from build123d import *

# Parameters (mm, degrees)
SKETCH1_R           = 125
SKETCH1_R_2         = 120
BOSS_EXTRUDE1_DEPTH = 10
SKETCH2_R           = 2.5
BOSS_EXTRUDE2_DEPTH = 100
SKETCH3_R           = 125
SKETCH3_R_2         = 120
BOSS_EXTRUDE3_DEPTH = 10
SKETCH4_R           = 2.5
BOSS_EXTRUDE4_DEPTH = 100
SKETCH5_R           = 125
SKETCH5_R_2         = 120
BOSS_EXTRUDE5_DEPTH = 10
SKETCH6_R           = 2.5
BOSS_EXTRUDE6_DEPTH = 100
SKETCH7_R           = 125
SKETCH7_R_2         = 120
BOSS_EXTRUDE7_DEPTH = 10
SKETCH8_R           = 2.5
BOSS_EXTRUDE8_DEPTH = 100
SKETCH9_R           = 125
SKETCH9_R_2         = 120
BOSS_EXTRUDE9_DEPTH = 10


with BuildPart() as part:
    # Sketch1 → Boss-Extrude1 (new body)
    with BuildSketch(Plane(origin=(0, 0, 0), x_dir=(1, 0, 0), z_dir=(0, 1, 0))):
        with Locations(Location((0, 0, 0), (0, 0, 270))):
            Circle(SKETCH1_R)
        with Locations(Location((0, 0, 0), (0, 0, 270))):
            Circle(SKETCH1_R_2, mode=Mode.SUBTRACT)
    extrude(amount=BOSS_EXTRUDE1_DEPTH)

    # Sketch2 → Boss-Extrude2 (add)
    with BuildSketch(Plane(origin=(0, 10, 0), x_dir=(1, 0, 0), z_dir=(0, 1, 0))):
        with Locations(Location((0, 122.5, 0), (0, 0, 270))):
            Circle(SKETCH2_R)
        with Locations(Location((106.088111964, 61.25, 0), (0, 0, 30))):
            Circle(SKETCH2_R)
        with Locations(Location((106.088111964, -61.25, 0), (0, 0, 150))):
            Circle(SKETCH2_R)
        with Locations(Location((0, -122.5, 0), (0, 0, 270))):
            Circle(SKETCH2_R)
        with Locations(Location((-106.088111964, -61.25, 0), (0, 0, 30))):
            Circle(SKETCH2_R)
        with Locations(Location((-106.088111964, 61.25, 0), (0, 0, 150))):
            Circle(SKETCH2_R)
    extrude(amount=BOSS_EXTRUDE2_DEPTH)

    # Sketch3 → Boss-Extrude3 (add)
    with BuildSketch(Plane(origin=(0, 110, 0), x_dir=(1, 0, 0), z_dir=(0, 1, 0))):
        with Locations(Location((0, 0, 0), (0, 0, 270))):
            Circle(SKETCH3_R)
        with Locations(Location((0, 0, 0), (0, 0, 270))):
            Circle(SKETCH3_R_2, mode=Mode.SUBTRACT)
    extrude(amount=BOSS_EXTRUDE3_DEPTH)

    # Sketch4 → Boss-Extrude4 (add)
    with BuildSketch(Plane(origin=(0, 120, 0), x_dir=(1, 0, 0), z_dir=(0, 1, 0))):
        with Locations(Location((0, 122.5, 0), (0, 0, 90))):
            Circle(SKETCH4_R)
        with Locations(Location((106.088111964, 61.25, 0), (0, 0, 30))):
            Circle(SKETCH4_R)
        with Locations(Location((106.088111964, -61.25, 0), (0, 0, 150))):
            Circle(SKETCH4_R)
        with Locations(Location((0, -122.5, 0), (0, 0, 90))):
            Circle(SKETCH4_R)
        with Locations(Location((-106.088111964, -61.25, 0), (0, 0, 30))):
            Circle(SKETCH4_R)
        with Locations(Location((-106.088111964, 61.25, 0), (0, 0, 150))):
            Circle(SKETCH4_R)
    extrude(amount=BOSS_EXTRUDE4_DEPTH)

    # Sketch5 → Boss-Extrude5 (add)
    with BuildSketch(Plane(origin=(0, 220, 0), x_dir=(1, 0, 0), z_dir=(0, 1, 0))):
        with Locations(Location((0, 0, 0), (0, 0, 270))):
            Circle(SKETCH5_R)
        with Locations(Location((0, 0, 0), (0, 0, 270))):
            Circle(SKETCH5_R_2, mode=Mode.SUBTRACT)
    extrude(amount=BOSS_EXTRUDE5_DEPTH)

    # Sketch6 → Boss-Extrude6 (add)
    with BuildSketch(Plane(origin=(0, 230, 0), x_dir=(1, 0, 0), z_dir=(0, 1, 0))):
        with Locations(Location((0, 122.5, 0), (0, 0, 90))):
            Circle(SKETCH6_R)
        with Locations(Location((106.088111964, 61.25, 0), (0, 0, 30))):
            Circle(SKETCH6_R)
        with Locations(Location((106.088111964, -61.25, 0), (0, 0, 150))):
            Circle(SKETCH6_R)
        with Locations(Location((0, -122.5, 0), (0, 0, 90))):
            Circle(SKETCH6_R)
        with Locations(Location((-106.088111964, -61.25, 0), (0, 0, 30))):
            Circle(SKETCH6_R)
        with Locations(Location((-106.088111964, 61.25, 0), (0, 0, 150))):
            Circle(SKETCH6_R)
    extrude(amount=BOSS_EXTRUDE6_DEPTH)

    # Sketch7 → Boss-Extrude7 (add)
    with BuildSketch(Plane(origin=(0, 330, 0), x_dir=(1, 0, 0), z_dir=(0, 1, 0))):
        with Locations(Location((0, 0, 0), (0, 0, 270))):
            Circle(SKETCH7_R)
        with Locations(Location((0, 0, 0), (0, 0, 270))):
            Circle(SKETCH7_R_2, mode=Mode.SUBTRACT)
    extrude(amount=BOSS_EXTRUDE7_DEPTH)

    # Sketch8 → Boss-Extrude8 (add)
    with BuildSketch(Plane(origin=(0, 340, 0), x_dir=(1, 0, 0), z_dir=(0, 1, 0))):
        with Locations(Location((0, 122.5, 0), (0, 0, 90))):
            Circle(SKETCH8_R)
        with Locations(Location((106.088111964, 61.25, 0), (0, 0, 30))):
            Circle(SKETCH8_R)
        with Locations(Location((106.088111964, -61.25, 0), (0, 0, 150))):
            Circle(SKETCH8_R)
        with Locations(Location((0, -122.5, 0), (0, 0, 90))):
            Circle(SKETCH8_R)
        with Locations(Location((-106.088111964, -61.25, 0), (0, 0, 30))):
            Circle(SKETCH8_R)
        with Locations(Location((-106.088111964, 61.25, 0), (0, 0, 150))):
            Circle(SKETCH8_R)
    extrude(amount=BOSS_EXTRUDE8_DEPTH)

    # Sketch9 → Boss-Extrude9 (add)
    with BuildSketch(Plane(origin=(0, 440, 0), x_dir=(1, 0, 0), z_dir=(0, 1, 0))):
        with Locations(Location((0, 0, 0), (0, 0, 270))):
            Circle(SKETCH9_R)
        with Locations(Location((0, 0, 0), (0, 0, 270))):
            Circle(SKETCH9_R_2, mode=Mode.SUBTRACT)
    extrude(amount=BOSS_EXTRUDE9_DEPTH)


solid = part.part
The listing builds one solid part. Answer for the finished solid, in the listing's coordinates (mm). Give positions to 0.01 mm unless a question says otherwise; leave off trailing zeros. Loops run counter-clockwise (first coordinate to the right, second up) from the corner with the lowest first, then second, coordinate; pieces in that order, holes last. Notation, with made-up numbers: (75.25, 84) - (103.25, 84) arc R20 ccw to (103.25, 101) - close; hole circle Ø4 at (-21, 18). An arc over 180 degrees is marked (long way). Write each question's results on one line, items separated by ' | '.
1. Find section B-B, the plane z = 0. Count the separate pieces of the cut face and the enclosed holes in it, then the cut area to 3 significant figures.
Resolved:
separate pieces: 10 | enclosed holes: 0 | area: 500 mm^2
2. Find section A-A, the plane y = 395. Write down the section's boundary in (x, z).
Resolved:
outline: circle Ø5 at (-106.09, -61.25); circle Ø5 at (-106.09, 61.25); circle Ø5 at (0, -122.5); circle Ø5 at (0, 122.5); circle Ø5 at (106.09, -61.25); circle Ø5 at (106.09, 61.25)
3. Consider probe 1 along X at (y, z) = (225, 0); probe 2 along X at (y, z) = (355.5, 60.5); probe 3 along Z at (x, y) = (1, 70.5). Determine where each line is inside the solid, lowest interval first. Write a range as from..to.
Resolved:
probe 1: x = -125..-120, 120..125 | probe 2: x = -108.47..-103.7, 103.7..108.47 | probe 3: z = -124.79..-120.21, 120.21..124.79
4. For a pull along Z with two mould halves and no side action, classify faces 1 (the face through (5.276, 334.93, -119.884)), 2 (the face through (112, 450, -47)), 3 (the face through (5.5, 114.93, -124.88)) as +Z half, -Z half, draft (parallel to the pull), parting line (faces both ways), or undercut.
Resolved:
face 1: undercut | face 2: draft | face 3: parting line
5. Find section C-C, the plane y = 115. Write down the section's boundary in (x, z), then the cut area to 3 significant figures.
Resolved:
outline: circle Ø250 at (0, 0); hole circle Ø240 at (0, 0) | area: 3,850 mm^2
6. Flat-ended cylindrical pins translate along their axes: P1, Ø6.5, axis at x = -114.5, z = 13, coming from the +Y side; P2, Ø12, axis at y = 344, z = 26.5, coming from the +X side. Find the tip coordinate at first contact, or state that the pin passes through.
Resolved:
P1: passes through | P2: stops at x = 123.04
